Autodesk Inventor part; units mm, degrees
ref_plane "YZ Plane" through (0, 0, 0) normal (1, 0, 0) x (0, 1, 0)
ref_plane "XZ Plane" through (0, 0, 0) normal (0, 1, 0) x (-1, 0, 0)
ref_plane "XY Plane" through (0, 0, 0) normal (0, 0, 1) x (1, 0, 0)
sketch "Sketch1" plane through (0, 0, 0) normal (0, 0, 1) x (1, 0, 0)
  circle A0 centre (0, 0) radius 7.4
  dimension "d0" = 14.8
extrude "Extrusion1" add sketch "Sketch1" along normal blind 40
sketch "Sketch2" plane through (0, 0, 40) normal (0, 0, 1) x (1, 0, 0)
  line L0 (0, 0) -> (-4.9, 0)
  line L1 (0, 0) -> (4.9, 0)
  line L2 (0, 0) -> (0, 5.5)
  line L3 (0, 5.5) -> (-4.9, 5.5)
  line L4 (-4.9, 5.5) -> (-4.9, 0)
  line L5 (0, 5.5) -> (4.9, 5.5)
  line L6 (4.9, 5.5) -> (4.9, 0)
  line L7 (-4.9, 0) -> (-4.9, -10)
  line L8 (-4.9, -10) -> (4.9, -10)
  line L9 (4.9, -10) -> (4.9, 0)
  dimension "d3" = 4.9
  dimension "d4" = 4.9
  dimension "d5" = 5.5
  dimension "d6" = 10
extrude "Extrusion2" cut sketch "Sketch2" against normal blind 7.9
sketch "Sketch3" plane through (0, 0, 32.1) normal (0, 0, 1) x (1, 0, 0)
  line L0 (-4.9, -5.5453) -> (-4.9, 5.5)
  line L1 (-4.9, 5.5) -> (-4.9, 0.2)
  line L2 (-4.9, 0.2) -> (-4.1, 0.2)
  line L3 (-4.1, 0.2) -> (-4.1, -7.8)
  line L4 (-4.1, -7.8) -> (-4.9, -7.8)
  line L5 (-4.9, -7.8) -> (-4.9, 0.2)
  line L6 (4.9, 5.5) -> (4.9, -5.5453)
  line L7 (4.9, 5.5) -> (4.9, 0.2)
  line L8 (4.9, 0.2) -> (4.1, 0.2)
  line L9 (4.1, 0.2) -> (4.1, -7.8)
  line L10 (4.1, -7.8) -> (4.9, -7.8)
  line L11 (4.9, 0.2) -> (4.9, -7.8)
  point P0 (0, 0)
  dimension "d9" = 5.3
  dimension "d10" = 0.8
  dimension "d11" = 8
  dimension "d12" = 0.8
  dimension "d13" = 5.3
  dimension "d14" = 0.8
  dimension "d15" = 8
extrude "Extrusion3" cut sketch "Sketch3" against normal blind 5
sketch "Sketch4" plane through (-4.9, 5.5, 40) normal (0, -1, 0) x (1, 0, 0)
  line L0 (12.3, 0) -> (-2.5, 0)
  line L1 (6.9, 0) -> (2.9, 0)
  line L2 (4.9, 0) -> (4.9, -1.2)
  line L3 (4.9, -1.2) -> (6.9, -1.2)
  line L4 (6.9, -1.2) -> (6.9, 0)
  line L5 (4.9, -1.2) -> (2.9, -1.2)
  line L6 (2.9, -1.2) -> (2.9, 0)
  point P0 (4.9, -40)
  point P1 (9.8, 0)
  point P2 (0, 0)
  dimension "d18" = 1.2
  dimension "d19" = 2
  dimension "d20" = 2
extrude "Extrusion4" add sketch "Sketch4" along normal blind 2
sketch "Sketch5" plane through (0, 0, 0) normal (0, 1, 0) x (-1, 0, 0)
  line L0 (-7.4, 0) -> (-7.4, 40)
  line L1 (-7.4, 40) -> (-7.4, 0)
  line L2 (-7.4, 20) -> (7.4, 20)
  line L3 (7.4, 0) -> (7.4, 40)
  circle A0 centre (0, 20) radius 5
  point P0 (0, 0)
  dimension "d23" = 10
extrude "Extrusion5" add sketch "Sketch5" against normal blind 80
ref_plane "Work Plane1" through (4.9, -5.5453, 27.1) normal (0, -1, 0) x (1, 0, 0)
sketch "Sketch7" plane through (0, 0, 0) normal (0, 0, -1) x (-1, 0, 0)
  circle A0 centre (0, 0) radius 3
  dimension "d26" = 6
ref_plane "Work Plane2" through (0, 0, 0) normal (-1, 0, 0) x (0, 0, -1)
sketch "Sketch8" plane through (0, 0, 0) normal (-1, 0, 0) x (0, 0, -1)
  line L0 (0, -7.4) -> (0, 7.4)
  circle A0 centre (0, 7.4) radius 7.4
  point P0 (0, 0)
sweep "Sweep1" cut profiles "Sketch7" path "Sketch8" path curves A0
equation "\"BendRadius\" = Thickness"
equation "\"BendReliefWidth\" = Thickness"
equation "\"BendReliefDepth\" = 0.5 * Thickness"
equation "\"CornerReliefSize\" = 4 * Thickness"
equation "\"MinimumRemnant\" = 2 * Thickness"
equation "\"TransitionRadius\" = BendRadius"
equation "\"JacobiRadiusSize\" = BendRadius"
equation "\"GapSize\" = Thickness"
properties part number "rotor1"
CAD build for the part. Positions are in the model's coordinates, mm. A direction names the side the tool comes from. Round coordinates to 2 decimals unless told otherwise and drop trailing zeros. Write each loop counter-clockwise with the first axis right and the second up, starting at its lowest first coordinate (ties: lowest second). Pieces come first, ordered by that corner, then holes. Notation, with made-up numbers: M 39.25,-2.75 L 86.25,-2.75 A23 cw 86.25,30.25 Z; hole C 20.5,-20 d6. An arc over 180 degrees is marked long. Use a Markdown table: item, result. Add a question column.
1. Slice it at C-C on y = -8.5. Give the cut face in (x, z), then the cut area to 3 significant figures.
2. Pull direction Z, two halves, no side cores. Call faces 1 (the face through (1.08, -42.21, 15.12)), 2 (the face through (0, -80, 20)), 3 (the face through (0, 5, 38.8)): released by +Z, released by -Z, zero draft, split by the parting line, or undercut.
3. Drill centre lines: probe 1 along X at (y, z) = (-70, 21); probe 2 along X at (y, z) = (-10, 24); probe 3 along X at (y, z) = (1, 5.5). Where is each one in solid material? Low to high.
4. Flat gauge pins, fed straight in: P1, Ø1.5, axis at x = -1, z = 26, coming from the -Y side; P2, Ø4, axis at x = 1, y = -46.5, coming from the -Z side; P3, Ø4, axis at y = -3, z = 29, coming from the +X side. Where does each tip first touch, or does it go through?
5. Slice it at B-B on z = 31. Give the cut face in (x, y), then the cut area to 3 significant figures.
6. Slice it at A-A on x = 0. Give the cut face in (y, z).
7. 3-axis set-ups, long thin cutter, end or side, ignore diameter. For faces 4 (the face through (4.1, -3, 30)), 5 (the face through (1, 4, 40)): which of +Z, -Z, +X, -X, +Y, -Y reach the whole face in a straight line?
8. Slice it at D-D on x = -6. Give the cut face in (y, z), then the cut area to 3 significant figures.
Reply:
| question | item | result |
|---|---|---|
| 1 | outline | C 0,20 d10 |
| 1 | area | 78.5 mm^2 |
| 2 | face 1 | split by the parting line |
| 2 | face 2 | zero draft |
| 2 | face 3 | undercut |
| 3 | probe 1 | x = -4.9 to 4.9 |
| 3 | probe 2 | x = -3 to 3 |
| 3 | probe 3 | x = -7.33 to -1.42, 1.42 to 7.33 |
| 4 | P1 | stops at y = -7.4 |
| 4 | P2 | stops at z = 15 |
| 4 | P3 | stops at x = 7.33 |
| 5 | outline | M -4.9,-5.55 L -4.9,0.2 L -4.1,0.2 L -4.1,-6.16 A7.4 ccw 4.1,-6.16 L 4.1,0.2 L 4.9,0.2 L 4.9,-5.55 A7.4 ccw long Z |
| 5 | area | 162 mm^2 |
| 6 | outline | M -80,15 L -7.4,15 L -7.4,10.4 A10.4 cw 3,0 L 7.4,0 L 7.4,40 L 3.5,40 L 3.5,38.8 L 5.5,38.8 L 5.5,32.1 L -7.4,32.1 L -7.4,25 L -80,25 Z; M -7.4,0 L -3,0 A4.4 ccw -7.4,4.4 Z |
| 7 | face 4 | +Z, -Y |
| 7 | face 5 | +Z, +X, -X, +Y, -Y |
| 8 | outline | M -4.33,0 L 4.33,0 L 4.33,40 L -4.33,40 Z |
| 8 | area | 347 mm^2 |
